Could you check a few things on this drawing? It's one solid part, dimensions in mm from its lowest x, y, z. Give positions to 0.01 mm unless a question says otherwise; leave off trailing zeros. Order: outer loops, then holes, each group sorted by start corner. A loop starts at its lowest first (then second) coordinate and runs counter-clockwise, first axis right, second up.
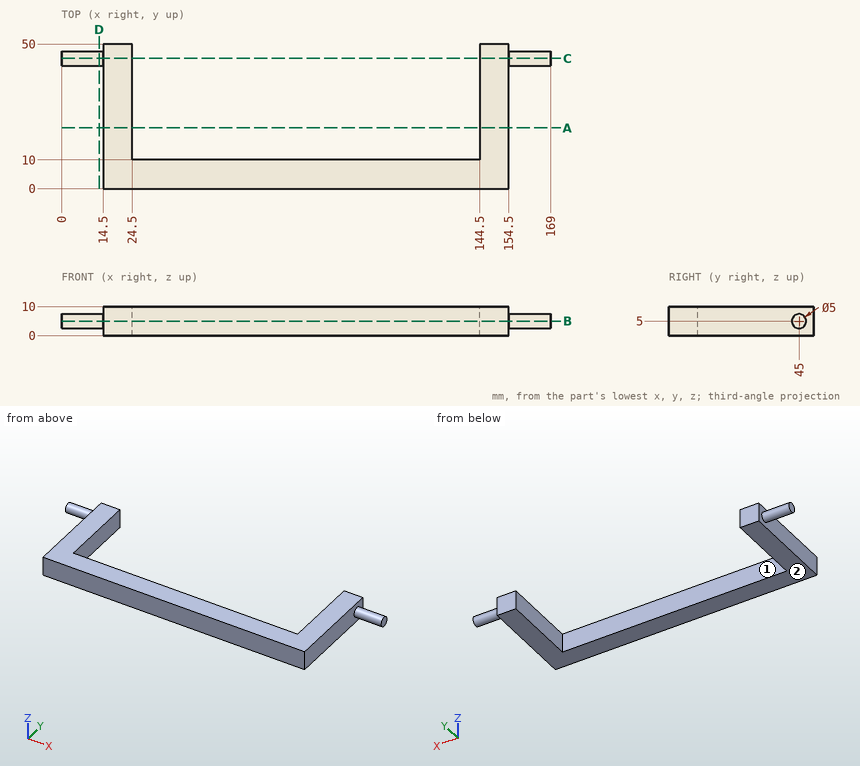
Q1. If we section it at B-B on z = 5: List the corners of the cut face in (x, y) for me.
Filled sheet:
outline: (0, 42.5) - (14.5, 42.5) - (14.5, 0) - (154.5, 0) - (154.5, 42.5) - (169, 42.5) - (169, 47.5) - (154.5, 47.5) - (154.5, 50) - (144.5, 50) - (144.5, 10) - (24.5, 10) - (24.5, 50) - (14.5, 50) - (14.5, 47.5) - (0, 47.5) - close
Q2. I need wall thicknesses on L1, parallel to X at y = 37, z = 5.5; L2, parallel to Y at x = 32.5, z = 2.25; L3, parallel to X at y = 7, z = 0.5. Which ranges of each line are inside material? Lowest first, please.
Filled sheet:
L1: x = 14.5 to 24.5, 144.5 to 154.5
L2: y = 0 to 10
L3: x = 14.5 to 154.5
Q3. Thinking about a two-plate mould opening in X: for the marked faces 1 and 2, which applies, released by +X, released by -X, zero draft, split by the parting line, or undercut?
Filled sheet:
face 1: undercut
face 2: zero draft
Q4. I'm going to push flat-ended pins straight in: P1, Ø2, axis at y = 45, z = 7, coming from the -X side; P2, Ø6, axis at x = 141, z = 2, coming from the +Y side; P3, Ø3, axis at y = 29.5, z = 4, coming from the -X side; P4, Ø3, axis at y = 12.5, z = 7.5, coming from the +X side. Where does each tip first touch, or does it pass through?
Filled sheet:
P1: stops at x = 0
P2: stops at y = 10
P3: stops at x = 14.5
P4: stops at x = 154.5
Q5. If we section it at C-C on y = 45: List the corners of the cut face in (x, z) for me.
Filled sheet:
outline: (0, 2.5) - (14.5, 2.5) - (14.5, 0) - (24.5, 0) - (24.5, 10) - (14.5, 10) - (14.5, 7.5) - (0, 7.5) - close; (144.5, 0) - (154.5, 0) - (154.5, 2.5) - (169, 2.5) - (169, 7.5) - (154.5, 7.5) - (154.5, 10) - (144.5, 10) - close
Q6. If we section it at D-D on x = 13: List the corners of the cut face in (y, z) for me.
Filled sheet:
outline: circle Ø5 at (45, 5)
Q7. If we section it at A-A on y = 21: List the corners of the cut face in (x, z) for me, plus the area to 3 significant figures.
Filled sheet:
outline: (14.5, 0) - (24.5, 0) - (24.5, 10) - (14.5, 10) - close; (144.5, 0) - (154.5, 0) - (154.5, 10) - (144.5, 10) - close
area: 200 mm2
